Could you check a few things on this model? Use its own coordinates, in mm. A direction names the side the tool comes from. Give positions to 0.01 mm unless a question says otherwise; leave off trailing zeros. Write each loop counter-clockwise with the first axis right and the second up, starting at its lowest first coordinate (ties: lowest second). Pieces come first, ordered by that corner, then holes. Notation, with made-up numbers: (79, 6.5) -> (90, 6.5) arc R6 cw to (90, 16.5) -> close; hole circle Ø7 at (73, 68). An arc over 180 degrees is marked (long way). One line per question, with ' | ' between items.
from build123d import *

# Parameters (mm, degrees)
BOSS_EXTRU_1_DEPTH      = 54
ESQUISSE2_R             = 1.75
ENL_V_MAT_EXTRU_1_DEPTH = 55.465585465


with BuildPart() as part:
    # Esquisse1 → Boss.-Extru.1 (new body)
    with BuildSketch(Plane.XY):
        Polygon((-2.5, 0), (2.5, 0), (5.5, 3), (5.5, 3.5), (2.95, 3.5), (2.95, 4.5), (-2.95, 4.5), (-2.95, 3.5), (-5.5, 3.5), (-5.5, 3), align=None)
    extrude(amount=BOSS_EXTRU_1_DEPTH)

    # Esquisse2 → Enlèv. mat.-Extru.1 (cut, through all)
    with BuildSketch(Plane(origin=(0, 4.5, 0), x_dir=(1, 0, 0), z_dir=(0, 1, 0))):
        with Locations(Location((0, -7, 0), (0, 0, 270))):
            Circle(ESQUISSE2_R)
        with Locations(Location((0, -47, 0), (0, 0, 90))):
            Circle(ESQUISSE2_R)
    extrude(amount=-ENL_V_MAT_EXTRU_1_DEPTH, mode=Mode.SUBTRACT)


solid = part.part
Q1. Imagine slicing it at A-A on x = 0. Please give me the cut outline in (y, z).
Answer below:
outline: (0, 0) -> (4.5, 0) -> (4.5, 5.25) -> (0, 5.25) -> close; (0, 8.75) -> (4.5, 8.75) -> (4.5, 45.25) -> (0, 45.25) -> close; (0, 48.75) -> (4.5, 48.75) -> (4.5, 54) -> (0, 54) -> close
Q2. Imagine slicing it at D-D on z = 30.5. Please give me the cut outline in (x, y).
Answer below:
outline: (-5.5, 3) -> (-2.5, 0) -> (2.5, 0) -> (5.5, 3) -> (5.5, 3.5) -> (2.95, 3.5) -> (2.95, 4.5) -> (-2.95, 4.5) -> (-2.95, 3.5) -> (-5.5, 3.5) -> close
Q3. If we mould it in two halves opening along Z, with no side actions, what happens to faces 1 (the cylindrical face through (0.526, 2.282, 8.669)), 2 (the flat face through (0, 2, 0)), 3 (the flat face through (-4, 1.5, 26.6))? For each: +Z half, -Z half, draft (parallel to the pull), parting line (faces both ways), or undercut.
Answer below:
face 1: undercut | face 2: -Z half | face 3: draft
Q4. Imagine slicing it at C-C on y = 1.15. Please give me the cut outline in (x, z), and give its area (3 significant figures).
Answer below:
outline: (-3.65, 0) -> (3.65, 0) -> (3.65, 54) -> (-3.65, 54) -> close; hole circle Ø3.5 at (0, 7); hole circle Ø3.5 at (0, 47) | area: 375 mm^2
Q5. On a 3-axis mill with a long thin cutter (end or side, diameter ignored), from which of +Z, -Z, +X, -X, +Y, -Y can I reach the whole of each face in a straight line? I mean faces 4 (the flat face through (2.95, 4, 27)), 5 (the flat face through (0, 4.5, 27)), 6 (the flat face through (-4, 3.5, 27)). Say none if no direction works.
Answer below:
face 4: +Z, -Z, +X, +Y | face 5: +Z, -Z, +X, -X, +Y | face 6: +Z, -Z, -X, +Y
Q6. Imagine slicing it at B-B on z = 47. Please give me the cut outline in (x, y).
Answer below:
outline: (-5.5, 3) -> (-2.5, 0) -> (-1.75, 0) -> (-1.75, 4.5) -> (-2.95, 4.5) -> (-2.95, 3.5) -> (-5.5, 3.5) -> close; (1.75, 0) -> (2.5, 0) -> (5.5, 3) -> (5.5, 3.5) -> (2.95, 3.5) -> (2.95, 4.5) -> (1.75, 4.5) -> close
Q7. Will these pins go through, and if not, where does the flat tip stop? pin 1 (1.3 mm diameter, centred on x = -5, z = 23, fed in from +Y); pin 2 (0.5 mm diameter, centred on y = 4, z = 22, fed in from +X).
Answer below:
pin 1: stops at y = 3.5 | pin 2: stops at x = 2.95
Q8. If I drill on line 1 along X through (y, z) = (3.3, 7); line 2 along Z through (x, y) = (-1.5, 0.55); line 3 along X through (y, z) = (4.25, 39), over which ranges is the centre line in solid material (lowest first)?
Answer below:
line 1: x = -5.5 to -1.75, 1.75 to 5.5 | line 2: z = 0 to 6.1, 7.9 to 46.1, 47.9 to 54 | line 3: x = -2.95 to 2.95
